Design review of the part shown in the three views and the two pictorial views. Dimensions are in mm from the part's minimum x, y and z. A direction names the side the tool comes from. Coordinates: 2 decimals unless noted, no trailing zeros. Loops run counter-clockwise (first coordinate to the right, second up) from the corner with the lowest first, then second, coordinate; pieces in that order, holes last.
Q1. For P1, Ø1, axis at x = 5, y = 22.5, coming from the -Z side; P2, Ø12, axis at x = 11.5, y = 14, coming from the -Z side, all flat-tipped, find the tip position at first contact; note any pin that passes through.
Q2. Add section A-A on y = 15.25. Give the boundary of the cut face in (x, z) (1 decimal).
Q3. Add section B-B on z = 87.5. Give the boundary of the cut face in (x, y) (1 decimal).
Q4. Machinability: for the marked faces 4 and 5, which of the approach directions +Z, -Z, +X, -X, +Y, -Y give a long, thin tool a straight path to every point of the face, cutting with its end or side? Answer none if there is none.
Q5. Add section C-C on x = 19.75. Give the boundary of the cut face in (y, z) (1 decimal), and give its area (3 significant figures).
Q6. Draft analysis for pull direction Y (two halves, no side actions). For the marked faces 1, 2 and 3, state which applies: released by +Y, released by -Y, zero draft, split by the parting line, or undercut.
Q7. Wall thickness on probe 1 along X at (y, z) = (3.75, 12.5) (1 decimal); probe 2 along Z at (x, y) = (19.5, 24.75): over which ranges is each line inside the solid? List them lowest first.
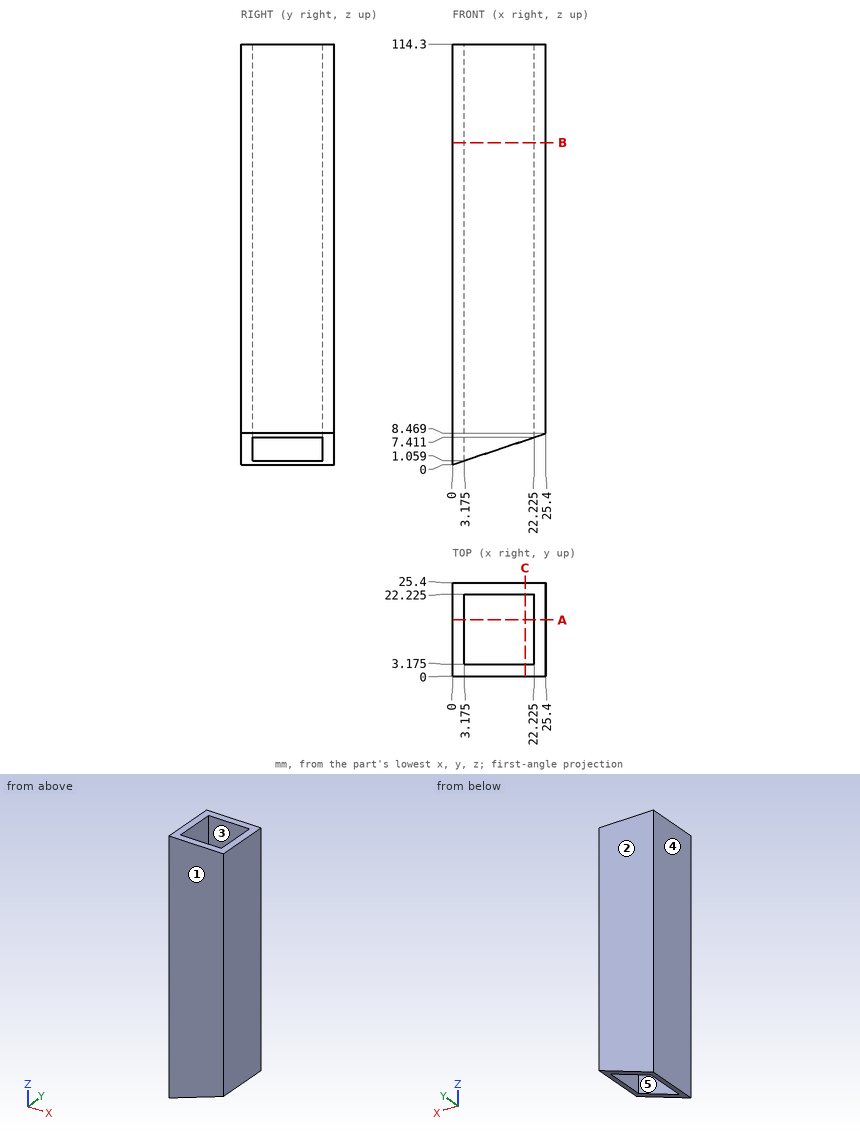
Entries:
1. P1: stops at z = 1.5
1. P2: passes through
2. outline: (0, 0) - (3.2, 1.1) - (3.2, 114.3) - (0, 114.3) - close; (22.2, 7.4) - (25.4, 8.5) - (25.4, 114.3) - (22.2, 114.3) - close
3. outline: (0, 0) - (25.4, 0) - (25.4, 25.4) - (0, 25.4) - close; hole (3.2, 3.2) - (22.2, 3.2) - (22.2, 22.2) - (3.2, 22.2) - close
4. face 4: +Z, -Z, -X, +Y, -Y
4. face 5: +Z, -Z
5. outline: (0, 6.6) - (3.2, 6.6) - (3.2, 114.3) - (0, 114.3) - close; (22.2, 6.6) - (25.4, 6.6) - (25.4, 114.3) - (22.2, 114.3) - close
5. area: 684 mm2
6. face 1: released by -Y
6. face 2: released by +Y
6. face 3: undercut
7. probe 1: x = 0 to 3.2, 22.2 to 25.4
7. probe 2: z = 6.5 to 114.3
